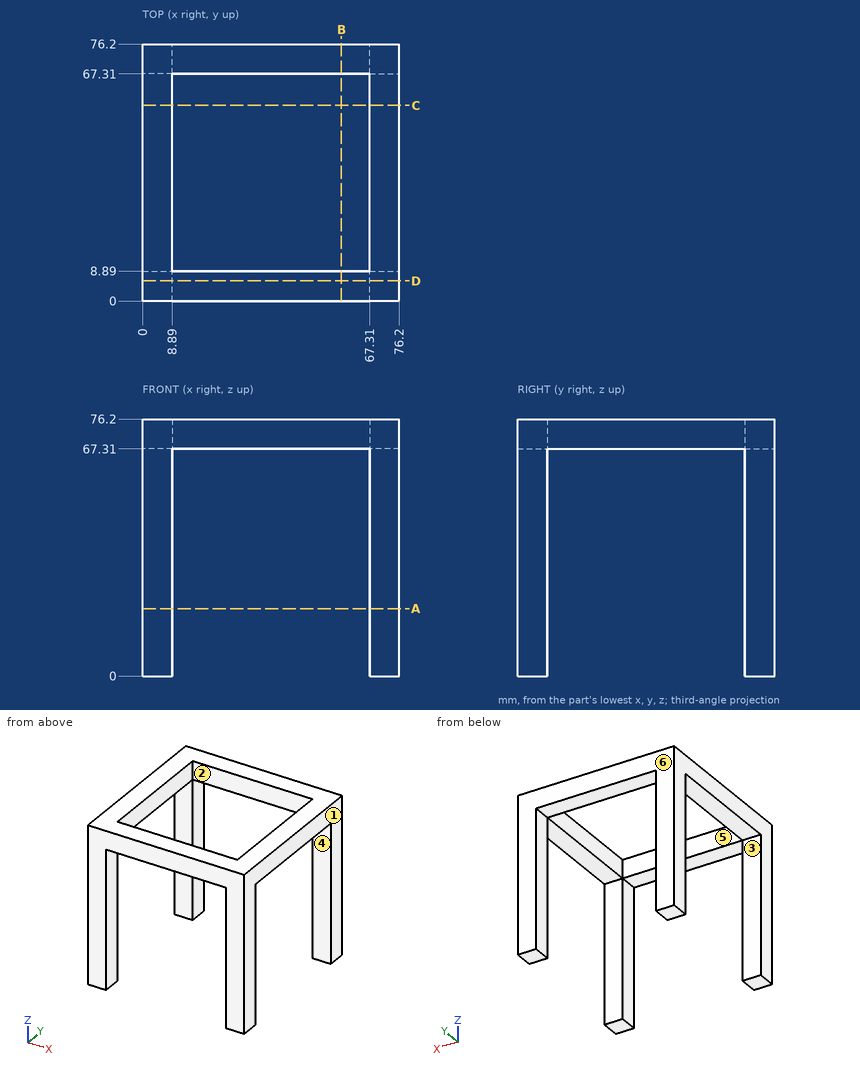
The figure shows three views and two pictorial views of one solid part (mm, origin at its lowest corner). Answer the questions. A direction names the side the tool comes from. Round coordinates to 2 decimals unless told otherwise and drop trailing zeros. Order: outer loops, then holes, each group sorted by start corner. A loop starts at its lowest first (then second) coordinate and runs counter-clockwise, first axis right, second up. Notation, with made-up numbers: (70.25, 31.5) -> (106.25, 31.5) arc R34 ccw to (106.25, 66.5) -> close; hole circle Ø1 at (-32.5, 42). An arc over 180 degrees is marked (long way). Put each result on its own line as item: value.
Q1. Section D-D, the plane y = 6 is taken. Write down the section's boundary in (x, z), and give its area (3 significant figures).
Results list:
outline: (0, 0) -> (8.89, 0) -> (8.89, 67.31) -> (67.31, 67.31) -> (67.31, 0) -> (76.2, 0) -> (76.2, 76.2) -> (0, 76.2) -> close
area: 1,870 mm^2
Q2. Consider line 1 along Y through (x, z) = (34, 67.5); line 2 along Z through (x, y) = (72, 22). Determine where each line is inside the solid, lowest interval first.
Results list:
line 1: 0 to 8.89, 67.31 to 76.2
line 2: 67.31 to 76.2
Q3. Section A-A, the plane z = 20 is taken. Write down the section's boundary in (x, y).
Results list:
outline: (0, 0) -> (8.89, 0) -> (8.89, 8.89) -> (0, 8.89) -> close; (0, 67.31) -> (8.89, 67.31) -> (8.89, 76.2) -> (0, 76.2) -> close; (67.31, 0) -> (76.2, 0) -> (76.2, 8.89) -> (67.31, 8.89) -> close; (67.31, 67.31) -> (76.2, 67.31) -> (76.2, 76.2) -> (67.31, 76.2) -> close
Q4. Which of the six approach directions +Z, -Z, +X, -X, +Y, -Y give full straight-line access (tool end or side, diameter ignored) to the marked faces 4, 5 and 6?
Results list:
face 4: -Z, +X, -X
face 5: +Z, -Z
face 6: +Z, -Z, +X, -X, +Y
Q5. Section B-B, the plane x = 59 is taken. Write down the section's boundary in (y, z).
Results list:
outline: (0, 67.31) -> (8.89, 67.31) -> (8.89, 76.2) -> (0, 76.2) -> close; (67.31, 67.31) -> (76.2, 67.31) -> (76.2, 76.2) -> (67.31, 76.2) -> close
Q6. Determine the mould class of the marked faces 1, 2 and 3 for opening direction X: pulls with the +X half, pulls with the -X half, needs draft (parallel to the pull), parting line crosses it, or undercut.
Results list:
face 1: pulls with the +X half
face 2: undercut
face 3: needs draft
Q7. This flat-tipped pin is pushed along its axis until it touches: P1, Ø7, axis at x = 3, y = 29.5, coming from the -Z side. Where does it stop, or does it pass through?
Results list:
P1: z = 67.31
